The model under review builds one solid part; all positions refer to its coordinate system, in mm. Face numbers are marked on the shaded views. A direction names the side the tool comes from. Coordinates: 2 decimals unless noted, no trailing zeros. Put each result on its own line as item: value. Start each with the question number.
Item 1: To check wall thickness, follow L1, parallel to Z at x = 12, y = 2; L2, parallel to X at y = 7.5, z = 13; L3, parallel to X at y = 8.5, z = 20. State the ranges of each line that lie inside material, in increasing order. Write a range as [from, to].
Item 2: Mouldability with a two-part tool opening along Z and no side actions: class the marked faces 3, 4 and 5 as pulls with the +Z half, pulls with the -Z half, needs draft (parallel to the pull), parting line crosses it, or undercut.
Item 3: Machinability: for the marked faces 1 and 2, which of the approach directions +Z, -Z, +X, -X, +Y, -Y give a long, thin tool a straight path to every point of the face, cutting with its end or side? Answer none if there is none.
Item 4: For pin 1 (3 mm diameter, centred on x = 16, y = 17.5, fed in from -Z); pin 2 (2 mm diameter, centred on x = 15.5, y = 6, fed in from -Z); pin 3 (5 mm diameter, centred on x = -5.5, y = 5.5, fed in from -Z); pin 4 (6 mm diameter, centred on y = 6.5, z = 25.5, fed in from -X), all flat-tipped, find the tip position at first contact; note any pin that passes through.
Item 5: Consider section A-A on y = 16.25. State how many separate pieces and enclosed holes the cut face has, then the cut area to 3 significant figures.
```python
from build123d import *

# Parameters (mm, degrees)
F1_DEPTH       = 25.4
F1_TAPER       = 2
F3_DEPTH       = 31.7510001
F5_DEPTH       = 20.6385001
F5_DEPTH_BACK  = 11.1135001
F6_W           = 6.096
F6_H           = 6.096
F7_DEPTH       = 6.35
F7_TAPER       = 2
F8_W           = 60.6717504561
F8_H           = 50.1286070794
F9_DEPTH       = 31.7510001
F10_W          = 37.0408929884
F10_H          = 41.4357688278
F11_DEPTH      = 11.1135001
F11_DEPTH_BACK = 20.6385001


with BuildPart() as f1:
    # F0 (on Front) → F1 (new body)
    with BuildSketch(Plane.XZ):
        Polygon((9.525, 31.75), (0, 31.75), (0, 20.6375), (-11.1125, 20.6375), (-11.1125, 11.1125), (0, 11.1125), (0, 0), (9.525, 0), (9.525, 11.1125), (20.6375, 11.1125), (20.6375, 20.6375), (9.525, 20.6375), align=None)
    extrude(amount=-F1_DEPTH, taper=F1_TAPER)

    # F2 (on Top) → F3 (cut, through all)
    with BuildSketch(Plane.XY):
        Polygon((2.8000508235, 25.4), (1.9685, 1.5875), (7.5565, 1.5875), (6.7249491765, 25.4), align=None)
    extrude(amount=F3_DEPTH, mode=Mode.SUBTRACT)

    # F4 (on Right) → F5 (cut, two sides)
    with BuildSketch(Plane.YZ) as f5_sk:
        Polygon((25.4, 17.8374491765), (1.5875, 18.669), (1.5875, 13.081), (25.4, 13.9125508235), align=None)
    extrude(amount=F5_DEPTH, mode=Mode.SUBTRACT)
    extrude(f5_sk.sketch, amount=-F5_DEPTH_BACK, mode=Mode.SUBTRACT)

    # F6 (on face) → F7 (join)
    with BuildSketch(Plane(origin=(0, 1.5875, 0), x_dir=(-1, 0, 0), z_dir=(0, 1, 0))):
        with Locations((-4.7625, 15.875)):
            Rectangle(F6_W, F6_H)
    extrude(amount=F7_DEPTH, taper=F7_TAPER)

    # F8 (on Top) → F9 (cut, through all)
    with BuildSketch(Plane.XY):
        with Locations((4.5310724527, 13.3044691756)):
            Rectangle(F8_W, F8_H)
        Polygon((20.6375, 0), (-11.1125, 0), (-1.9751491765, 25.4), (11.5001491765, 25.4), align=None, mode=Mode.SUBTRACT)
    extrude(amount=F9_DEPTH, mode=Mode.SUBTRACT)

    # F10 (on Right) → F11 (cut, two sides)
    with BuildSketch(Plane.YZ) as f11_sk:
        with Locations((11.8458718061, 15.7928168774)):
            Rectangle(F10_W, F10_H)
        Polygon((0, 0), (0, 31.75), (25.4, 22.6126491765), (25.4, 9.1373508235), align=None, mode=Mode.SUBTRACT)
    extrude(amount=-F11_DEPTH, mode=Mode.SUBTRACT)
    extrude(f11_sk.sketch, amount=F11_DEPTH_BACK, mode=Mode.SUBTRACT)


solid = f1.part
```
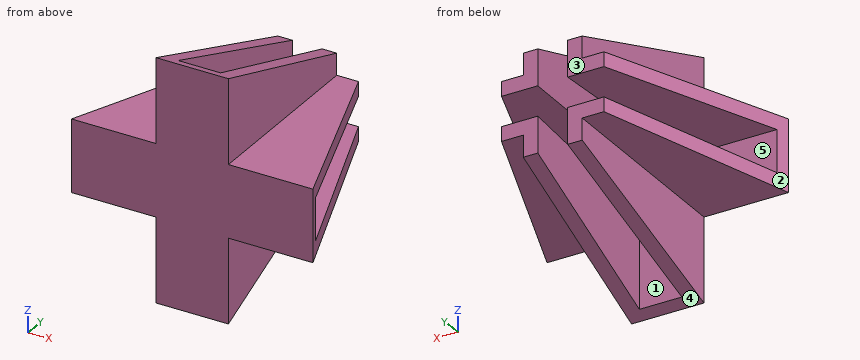
Report:
1. L1: [11.18, 13.1], [18.65, 20.57]
1. L2: [-8.41, 2.17], [7.35, 17.94]
1. L3: [-8.05, 2.21], [7.32, 17.58]
2. face 3: needs draft
2. face 4: pulls with the -Z half
2. face 5: undercut
3. face 1: -Z
3. face 2: +Z, -Z, -X, +Y
4. pin 1: through
4. pin 2: z = 11.29
4. pin 3: z = 11.22
4. pin 4: x = 0.12
5. separate pieces: 4
5. enclosed holes: 0
5. area: 104 mm²
